Read the model definition and answer for the solid it produces. Units are mm, in the model's axes. A direction names the side the tool comes from. Coordinates: 2 decimals unless noted, no trailing zeros. Write each loop counter-clockwise with the first axis right and the second up, starting at its lowest first coordinate (ties: lowest second). Pieces come first, ordered by that corner, then holes. Notation, with made-up numbers: (-23, 76.25) - (-15, 76.25) arc R7 ccw to (-15, 84.25) - close; hole circle Ø11 at (1.5, 35). An arc over 180 degrees is marked (long way). Use a Markdown table: item, result.
from build123d import *

# Parameters (mm, degrees)
SKETCH_W        = 203
SKETCH_H        = 153
SKETCH_W_2      = 163.5
SKETCH_H_2      = 98
PAD_DEPTH       = 2
SKETCH003_W     = 172
SKETCH003_H     = 111.5
POCKET001_DEPTH = 1
SKETCH002_W     = 22
SKETCH002_H     = 22
SKETCH002_W_2   = 15
SKETCH002_H_2   = 15
POCKET_DEPTH    = 1
SKETCH001_R     = 2.625
PAD001_DEPTH    = 5


with BuildPart() as part:
    # Sketch (on DatumPlane) → Pad (new body)
    with BuildSketch(Plane.XY.offset(-2)):
        Rectangle(SKETCH_W, SKETCH_H)
        Rectangle(SKETCH_W_2, SKETCH_H_2, mode=Mode.SUBTRACT)
    extrude(amount=PAD_DEPTH)

    # Sketch003 (on DatumPlane) → Pocket001 (cut)
    with BuildSketch(Plane.XY):
        with Locations((0, -3.75)):
            Rectangle(SKETCH003_W, SKETCH003_H)
    extrude(amount=-POCKET001_DEPTH, mode=Mode.SUBTRACT)

    # Sketch002 (on DatumPlane) → Pocket (cut)
    with BuildSketch(Plane.XY):
        with Locations((0, 64)):
            Rectangle(SKETCH002_W, SKETCH002_H)
        with Locations((0, -61.5)):
            Rectangle(SKETCH002_W_2, SKETCH002_H_2)
    extrude(amount=-POCKET_DEPTH, mode=Mode.SUBTRACT)

    # Sketch001 (on DatumPlane) → Pad001 (join)
    with BuildSketch(Plane.XY):
        with Locations((89, 64)):
            Circle(SKETCH001_R)
        with Locations((-89, 64)):
            Circle(SKETCH001_R)
        with Locations((-89, -64)):
            Circle(SKETCH001_R)
        with Locations((89, -64)):
            Circle(SKETCH001_R)
    extrude(amount=PAD001_DEPTH)


solid = part.part
(1) The mould has two halves that part along Y. Classify faces 1 (the cylindrical face through (-86.575, 62.995, 2.465)), 2 (the flat face through (-89, 64, 5)): pulls with the +Y half, pulls with the -Y half, needs draft (parallel to the pull), parting line crosses it, or undercut.
Report:
| item | result |
|---|---|
| face 1 | undercut |
| face 2 | needs draft |
(2) A cutting plane is placed at C-C, the plane z = 2.75. Write down the section's boundary in (x, y) (3 decimals).
Report:
| item | result |
|---|---|
| outline | circle Ø5.25 at (-89, -64); circle Ø5.25 at (-89, 64); circle Ø5.25 at (89, -64); circle Ø5.25 at (89, 64) |
(3) A cutting plane is placed at D-D, the plane y = 64. Write down the section's boundary in (x, z) (3 decimals).
Report:
| item | result |
|---|---|
| outline | (-101.5, -2) - (101.5, -2) - (101.5, 0) - (91.625, 0) - (91.625, 5) - (86.375, 5) - (86.375, 0) - (11, 0) - (11, -1) - (-11, -1) - (-11, 0) - (-86.375, 0) - (-86.375, 5) - (-91.625, 5) - (-91.625, 0) - (-101.5, 0) - close |
(4) A cutting plane is placed at B-B, the plane x = -77. Write down the section's boundary in (y, z), and give its area (3 significant figures).
Report:
| item | result |
|---|---|
| outline | (-76.5, -2) - (-49, -2) - (-49, -1) - (-59.5, -1) - (-59.5, 0) - (-76.5, 0) - close; (49, -2) - (76.5, -2) - (76.5, 0) - (52, 0) - (52, -1) - (49, -1) - close |
| area | 96.5 mm² |
(5) For faces 3 (the flat face through (89, 64, 5)), 4 (the flat face through (0, 64, -1)), determine the directions among +Z, -Z, +X, -X, +Y, -Y from which every point of the face is accessible in a straight line to the end or side of a thin tool.
Report:
| item | result |
|---|---|
| face 3 | +Z, +X, -X, +Y, -Y |
| face 4 | +Z |
(6) Straight lines are drawn through the part: L1, parallel to Y at x = 34.5, z = -0.25; L2, parallel to X at y = 22.5, z = -1.5; L3, parallel to X at y = -16.5, z = -0.5. For each, find the intervals that lie inside material, in ascending order.
Report:
| item | result |
|---|---|
| L1 | y = -76.5 to -59.5, 52 to 76.5 |
| L2 | x = -101.5 to -81.75, 81.75 to 101.5 |
| L3 | x = -101.5 to -86, 86 to 101.5 |
(7) A cutting plane is placed at A-A, the plane y = 6.5. Write down the section's boundary in (x, z).
Report:
| item | result |
|---|---|
| outline | (-101.5, -2) - (-81.75, -2) - (-81.75, -1) - (-86, -1) - (-86, 0) - (-101.5, 0) - close; (81.75, -2) - (101.5, -2) - (101.5, 0) - (86, 0) - (86, -1) - (81.75, -1) - close |
(8) Each of these flat-tipped pins is pushed along its axis until it touches: P1, Ø6.5, axis at x = -3.5, y = 63.5, coming from the +Z side; P2, Ø4, axis at y = 4.5, z = 1.5, coming from the -X side. Where does it stop, or does it pass through?
Report:
| item | result |
|---|---|
| P1 | stops at z = -1 |
| P2 | stops at x = -101.5 |
